Autodesk Inventor part; units mm, degrees
ref_plane "YZ Plane" through (0, 0, 0) normal (1, 0, 0) x (0, 1, 0)
ref_plane "XZ Plane" through (0, 0, 0) normal (0, 1, 0) x (-1, 0, 0)
ref_plane "XY Plane" through (0, 0, 0) normal (0, 0, 1) x (1, 0, 0)
sketch "Sketch1" plane through (0, 0, 0) normal (0, 1, 0) x (-1, 0, 0)
  line L0 (48.734, 45) -> (-48.734, 45)
  line L1 (12, -60.25) -> (-12, -60.25)
  line L2 (-12, -58) -> (12, -58)
  circle A0 centre (0, 0) radius 6
  circle A1 centre (-22.2662, -63.1919) radius 1.5
  circle A2 centre (-41.7906, 34.5) radius 1.5
  circle A3 centre (-60.7226, -28.3154) radius 1.5
  circle A4 centre (60.7226, -28.3154) radius 1.5
  circle A5 centre (-20, 41.5) radius 1.5
  circle A6 centre (41.7906, 34.5) radius 1.5
  circle A7 centre (20, 41.5) radius 1.5
  circle A8 centre (22.2662, -63.1919) radius 1.5
  arc A9 (12, -60.25) -> (12, -58) centre (12, -59.125) ccw
  arc A10 (-12, -58) -> (-12, -60.25) centre (-12, -59.125) ccw
  circle A11 centre (0, 0) radius 67 construction
  circle A12 centre (0, 0) radius 54.1913 construction
  line L3 (0, 0) -> (0, 45)
  arc A13 (-56.8563, 40.8333) -> (56.8563, 40.8333) centre (0, 0) ccw
  arc A14 (-48.734, 45) -> (-56.8563, 40.8333) centre (-48.734, 35) ccw
  arc A15 (56.8563, 40.8333) -> (48.734, 45) centre (48.734, 35) ccw
  line L4 (0, 0) -> (-70, 0)
  line L5 (0, 0) -> (60.7226, -28.3154) construction
  line L6 (0, 0) -> (67, 0)
  line L7 (0, 0) -> (41.7906, 34.5) construction
  line L8 (44.9375, 23.5) -> (65.9375, 23.5)
  line L9 (65.9375, 23.5) -> (65.9375, -23.5)
  line L10 (65.9375, -23.5) -> (44.9375, -23.5)
  line L11 (44.9375, -23.5) -> (44.9375, 23.5)
  line L12 (44.9375, 23.5) -> (65.9375, -23.5) construction
  line L13 (65.9375, 23.5) -> (44.9375, -23.5) construction
  circle A16 centre (36.5375, -9) radius 1
  circle A17 centre (36.5375, 9) radius 1
  circle A18 centre (16, -4.35) radius 1.5
  circle A19 centre (33.75, -51) radius 1.5
  circle A20 centre (-16, -4.35) radius 1.5
  circle A21 centre (-33.75, -51) radius 1.5
  line L14 (-44.9375, 23.5) -> (-65.9375, 23.5)
  line L15 (-65.9375, 23.5) -> (-65.9375, -23.5)
  line L16 (-65.9375, -23.5) -> (-44.9375, -23.5)
  line L17 (-44.9375, -23.5) -> (-44.9375, 23.5)
  circle A22 centre (-36.5375, -9) radius 1
  circle A23 centre (-36.5375, 9) radius 1
  line L18 (10, 38.5) -> (-10, 38.5)
  line L19 (-10, 38.5) -> (-10, 30.5)
  line L20 (-10, 30.5) -> (10, 30.5)
  line L21 (10, 30.5) -> (10, 38.5)
  line L22 (10, 38.5) -> (-10, 30.5) construction
  line L23 (-10, 38.5) -> (10, 30.5) construction
  line L24 (39, -25.5) -> (33, -25.5)
  line L25 (33, -25.5) -> (33, -36.5)
  line L26 (33, -36.5) -> (39, -36.5)
  line L27 (39, -36.5) -> (39, -25.5)
  circle A24 centre (36, -38.5) radius 1
  line L28 (39, -31) -> (33, -31)
  circle A25 centre (36, -23.5) radius 1
  circle A26 centre (40.817, -45.3318) radius 1.5
  circle A27 centre (-41.7906, 34.5) radius 1.5
  circle A28 centre (-40.817, -45.3318) radius 1.5
  line L29 (41.7906, 34.5) -> (41.7906, 39.5)
  line L30 (41.7906, 39.5) -> (57.7906, 39.5)
  line L31 (0, 0) -> (22.2662, -63.1919) construction
  circle A29 centre (60.7226, 28.3154) radius 1.5
  circle A30 centre (-60.7226, 28.3154) radius 1.5
  line L32 (40.817, -45.3318) -> (0, 0) construction
  line L33 (0, 0) -> (60.7226, 28.3154) construction
  point P0 (-5.9883, -61.0615)
  point P1 (55.4375, 0)
  point P2 (-65.9375, -23.5)
  point P3 (0, 34.5)
  point P4 (36, -36.5)
  point P5 (53.2983, 43.8976)
  point P6 (0, -6)
  dimension "d12" = 12
  dimension "d0" = 3
  dimension "d1" = 3
  dimension "d4" = 3
  dimension "d15" = 24
  dimension "d16" = 3
  dimension "d62" = 2.25
  dimension "d148" = 3.5
  dimension "d276" = 134
  dimension "d285" = 140
  dimension "d286" = 45
  dimension "d287" = 10
  dimension "d288" = 12
  dimension "d289" = 40
  dimension "d290" = 3.5
  dimension "d291" = 20
  dimension "d293" = 25
  dimension "d300" = 21
  dimension "d301" = 47
  dimension "d304" = 2
  dimension "d305" = 8.4
  dimension "d306" = 9
  dimension "d307" = 3
  dimension "d311" = 16
  dimension "d318" = 33.75
  dimension "d321" = 20
  dimension "d322" = 8
  dimension "d323" = 11
  dimension "d324" = 6
  dimension "d325" = 2
  dimension "d326" = 2
  dimension "d327" = 15
  dimension "d338" = 33
  dimension "d342" = 5
  dimension "d344" = 16
  dimension "d345" = 11
  dimension "d346" = 39.541
  dimension "d347" = 108.3827
  dimension "d348" = 19.41
  dimension "d350" = 61
  dimension "d351" = 48
  dimension "d352" = 3
  dimension "d353" = 4.35
  dimension "d354" = 51
  dimension "d355" = 25
  dimension "d356" = 58
  dimension "d358" = 65.9375
extrude "Extrusion1" add sketch "Sketch1" along normal blind 3 contours A15 A13 L8 L11 L6 A0 L3 L20 L21 L18 L0 | L3 L18 L19 L20 A0 L4 L17 L14 A13 A14 L0 | A13 L16 L17 L4 A0 L6 L11 L10
fillet "Fillet1" radius 2 1 edges at (65.9375, 1.5, 23.5)
fillet "Fillet2" radius 2 3 edges at (65.9375, 1.5, -23.5) (-65.9375, 1.5, -23.5) (-65.9375, 1.5, 23.5)
sketch "Sketch2" plane through (0, 3, 0) normal (0, 1, 0) x (1, 0, 0)
  circle A0 centre (60.7226, 28.3154) radius 1.5
  circle A1 centre (60.7226, -28.3154) radius 1.5
  line L0 (60.7226, 28.3154) -> (60.7226, -28.3154)
  line L1 (60.7226, -28.3154) -> (60.7226, -30.3154)
  line L2 (60.7226, -26.3154) -> (59.2226, -26.3154)
  line L3 (-48.734, -45) -> (48.734, -45)
  line L4 (0, -45) -> (0, 70)
  arc A2 (64.8917, 26.25) -> (-64.8917, 26.25) centre (0, 0) ccw
  line L5 (57.6226, -30.3154) -> (57.6226, -26.3154)
  line L6 (57.6226, -26.3154) -> (59.2226, -26.3154)
  line L7 (60.7226, -26.3154) -> (60.7226, -30.3154)
  line L8 (57.6226, -30.3154) -> (57.6226, -31.8154)
  line L9 (57.6226, -31.8154) -> (60.7226, -31.8154)
  line L10 (60.7226, -31.8154) -> (60.7226, -30.3154)
  line L11 (60.7226, -28.3154) -> (57.6226, -28.3154)
  line L12 (-70, 0) -> (70, 0)
  line L13 (60.7226, 28.3154) -> (60.7226, 30.3154)
  line L14 (60.7226, 26.3154) -> (59.2226, 26.3154)
  line L15 (57.6226, 30.3154) -> (57.6226, 26.3154)
  line L16 (57.6226, 26.3154) -> (59.2226, 26.3154)
  line L17 (60.7226, 26.3154) -> (60.7226, 30.3154)
  line L18 (57.6226, 30.3154) -> (57.6226, 31.8154)
  line L19 (57.6226, 31.8154) -> (60.7226, 31.8154)
  line L20 (60.7226, 31.8154) -> (60.7226, 30.3154)
  line L21 (-60.7226, -26.3154) -> (-59.2226, -26.3154)
  line L22 (-57.6226, -30.3154) -> (-57.6226, -26.3154)
  line L23 (-57.6226, -26.3154) -> (-59.2226, -26.3154)
  line L24 (-60.7226, -26.3154) -> (-60.7226, -30.3154)
  line L25 (-57.6226, -30.3154) -> (-57.6226, -31.8154)
  line L26 (-57.6226, -31.8154) -> (-60.7226, -31.8154)
  line L27 (-60.7226, -31.8154) -> (-60.7226, -30.3154)
  line L28 (-60.7226, -28.3154) -> (-57.6226, -28.3154)
  line L29 (-57.6226, 31.8154) -> (-60.7226, 31.8154)
  line L30 (-57.6226, 30.3154) -> (-57.6226, 31.8154)
  line L31 (-57.6226, 30.3154) -> (-57.6226, 26.3154)
  line L32 (-57.6226, 26.3154) -> (-59.2226, 26.3154)
  line L33 (-60.7226, 26.3154) -> (-59.2226, 26.3154)
  line L34 (-60.7226, 31.8154) -> (-60.7226, 30.3154)
  line L35 (-60.7226, 28.3154) -> (-60.7226, 30.3154)
  line L36 (-60.7226, 26.3154) -> (-60.7226, 30.3154)
  line L37 (-60.7226, 28.3154) -> (-57.6226, 28.3154)
  line L38 (60.7226, 28.3154) -> (57.6226, 28.3154)
  point P0 (60.7226, 26.8154)
  point P1 (60.7226, 29.8154)
  point P2 (60.7226, -29.8154)
  point P3 (60.7226, -26.8154)
  point P4 (60.7226, -26.3154)
  dimension "d363" = 1.5
  dimension "d365" = 4
  dimension "d366" = 1.5
  dimension "d367" = 3.1
  dimension "d368" = 1.6
extrude "Extrusion2" [suppressed]
properties part number "base_chasis_v5"
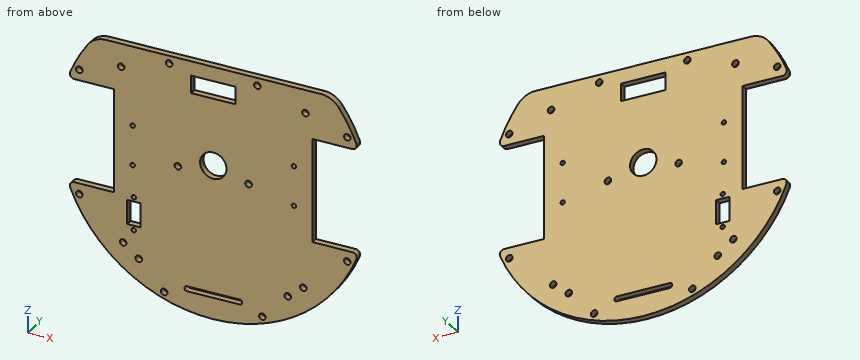
The listing builds one solid part. Answer for the finished solid, in the listing's coordinates (mm). Coordinates: 2 decimals unless noted, no trailing zeros. Write each loop counter-clockwise with the first axis right and the second up, starting at its lowest first coordinate (ties: lowest second). Pieces come first, ordered by that corner, then holes. Notation, with made-up numbers: M 18.25,54.25 L 34.25,54.25 A26 ccw 34.25,89.25 Z; hole C 12,-28 d8. An arc over 180 degrees is marked long. Use a Markdown table: item, result. Add a question column.
1. Given P1, Ø0.9, axis at y = 2, z = -28.5, coming from the -X side; P2, Ø2.5, axis at x = 16, z = -4.35, coming from the +Y side; P3, Ø1.5, axis at y = 1.5, z = -12.5, coming from the +X side; P4, Ø1, axis at x = 38, y = 1, coming from the -Z side, each flat-ended and moving along its own axis, determine where each tip first touches the part or whether it passes through.
2. Section C-C (x = 33.75) is taken. Give the vertices of the cut face in (y, z).
3. Section B-B (z = 0) is taken. Give the vertices of the cut face in (x, y).
4. Straight lines are drawn through the part: line 1 along X through (y, z) = (2.15, 0); line 2 along X through (y, z) = (2.4, -9.5); line 3 along X through (y, z) = (0.2, -63). For each, find the intervals that lie inside material, in ascending order. Write a range as [from, to].
5. Section A-A (x = 0) is taken. Give the vertices of the cut face in (y, z).
6. Section D-D (z = -51) is taken. Give the vertices of the cut face in (x, y).
Data:
| question | item | result |
|---|---|---|
| 1 | P1 | stops at x = -64.13 |
| 1 | P2 | passes through |
| 1 | P3 | stops at x = 44.94 |
| 1 | P4 | stops at z = -59.11 |
| 2 | outline | M 0,-61.33 L 3,-61.33 L 3,-52.5 L 0,-52.5 Z; M 0,-49.5 L 3,-49.5 L 3,45 L 0,45 Z |
| 3 | outline | M -44.94,0 L -6,0 L -6,3 L -44.94,3 Z; M 6,0 L 44.94,0 L 44.94,3 L 6,3 Z |
| 4 | line 1 | x = [-44.94, -6], [6, 44.94] |
| 4 | line 2 | x = [-44.94, -37.4], [-35.67, 35.67], [37.4, 44.94] |
| 4 | line 3 | x = [-30.51, -23.75], [-20.78, 20.78], [23.75, 30.51] |
| 5 | outline | M 0,-70 L 3,-70 L 3,-60.25 L 0,-60.25 Z; M 0,-58 L 3,-58 L 3,-6 L 0,-6 Z; M 0,6 L 3,6 L 3,30.5 L 0,30.5 Z; M 0,38.5 L 3,38.5 L 3,45 L 0,45 Z |
| 6 | outline | M -47.95,0 L -35.25,0 L -35.25,3 L -47.95,3 Z; M -32.25,0 L 32.25,0 L 32.25,3 L -32.25,3 Z; M 35.25,0 L 47.95,0 L 47.95,3 L 35.25,3 Z |
